Autodesk Inventor part; units mm, degrees
ref_plane "YZ Plane" through (0, 0, 0) normal (1, 0, 0) x (0, 1, 0)
ref_plane "XZ Plane" through (0, 0, 0) normal (0, 1, 0) x (-1, 0, 0)
ref_plane "XY Plane" through (0, 0, 0) normal (0, 0, 1) x (1, 0, 0)
sketch "Sketch1" plane through (0, 0, 0) normal (0, 0, 1) x (1, 0, 0)
  line L0 (0, 0) -> (0, 52)
  line L1 (0, 52) -> (3, 52)
  line L2 (3, 52) -> (3, 3)
  line L3 (3, 3) -> (52, 3)
  line L4 (52, 3) -> (52, 0)
  line L5 (52, 0) -> (0, 0)
  dimension "d0" = 3
  dimension "d1" = 3
  dimension "d2" = 52
  dimension "d3" = 52
extrude "Extrusion1" add sketch "Sketch1" along normal blind 50
sketch "Sketch2" plane through (3, 3, 0) normal (1, 0, 0) x (0, 0, -1)
  circle A0 centre (-25, 25) radius 8.8
  line L0 (0, 49) -> (-50, 49)
  line L1 (0, 0) -> (0, 49)
  circle A1 centre (-10.5, 25) radius 1.4515
  circle A2 centre (-39.5, 25) radius 1.4515
  point P0 (0, -3)
  dimension "d6" = 17.6
  dimension "d7" = 24
  dimension "d8" = 25
  dimension "d9" = 2.903
  dimension "d10" = 2.903
  dimension "d11" = 29
  dimension "d12" = 14.5
  dimension "d13" = 14.5
extrude "Extrusion2" cut sketch "Sketch2" against normal through all
sketch "Sketch3" plane through (3, 3, 0) normal (0, 1, 0) x (1, 0, 0)
  circle A0 centre (5.4515, -41.5485) radius 1.4515
  circle A1 centre (5.4515, -8.4515) radius 1.4515
  circle A2 centre (40.5485, -41.5485) radius 1.4515
  circle A3 centre (40.5485, -8.4515) radius 1.4515
  line L0 (49, -50) -> (0, -50)
  line L1 (49, 0) -> (0, 0)
  line L2 (49, 0) -> (49, -50)
  line L3 (-3, 0) -> (-3, -50)
  dimension "d16" = 2.903
  dimension "d17" = 2.903
  dimension "d18" = 2.903
  dimension "d19" = 2.903
  dimension "d20" = 7
  dimension "d21" = 7
  dimension "d22" = 7
  dimension "d23" = 7
  dimension "d24" = 7
  dimension "d25" = 7
  dimension "d26" = 7
  dimension "d27" = 7
extrude "Extrusion3" cut sketch "Sketch3" against normal through all
equation "\"BendRadius\" = Thickness"
equation "\"BendReliefWidth\" = Thickness"
equation "\"BendReliefDepth\" = 0.5 * Thickness"
equation "\"CornerReliefSize\" = 4 * Thickness"
equation "\"MinimumRemnant\" = 2 * Thickness"
equation "\"TransitionRadius\" = BendRadius"
equation "\"JacobiRadiusSize\" = BendRadius"
equation "\"GapSize\" = Thickness"
properties part number "dc motor clamp"
The model under review builds one solid part; all positions refer to its coordinate system, in mm. A direction names the side the tool comes from. Give positions to 0.01 mm unless a question says otherwise; leave off trailing zeros. Order: outer loops, then holes, each group sorted by start corner. A loop starts at its lowest first (then second) coordinate and runs counter-clockwise, first axis right, second up. Notation, with made-up numbers: M 62,-8.5 L 82,-8.5 A3 cw 82,-4.5 Z; hole C 39,-39 d7. An arc over 180 degrees is marked long. Answer in a Markdown table with one row per item. Add a question column.
1. Add section C-C on x = 8.5. State the section outline as (y, z) points.
2. For pin 1 Ø2 at (x, z) = (12.5, 20) entering from +Y; pin 2 Ø1.7 at (y, z) = (28, 10.5) entering from -X; pin 3 Ø5 at (y, z) = (40, 43.5) entering from +X, all flat-tipped, find the tip position at first contact; note any pin that passes through.
3. Add section D-D on z = 47. State the section outline as (x, y) points.
4. Mouldability with a two-part tool opening along X and no side actions: class faces 1 (the flat face through (0, 20, 19)), 2 (the cylindrical face through (42.479, 1.521, 40.568)), 3 (the flat face through (26, 0, 25)), 4 (the flat face through (3, 39, 25)) as released by +X, released by -X, zero draft, split by the parting line, or undercut.
5. Machinability: for faces 5 (the flat face through (27, 3, 25)), 6 (the cylindrical face through (1.52, 28.98, 40.57)), which of the approach directions +Z, -Z, +X, -X, +Y, -Y give a long, thin tool a straight path to every point of the face, cutting with its end or side? Answer none if there is none.
6. To check wall thickness, follow line 1 along X through (y, z) = (11, 29); line 2 along Y through (x, z) = (1, 25). State the ranges of each line that lie inside material, in increasing order.
7. Add section A-A on z = 25. State the section outline as (x, y) points.
8. Add section B-B on y = 20. State the section outline as (x, z) points.
The answers:
| question | item | result |
|---|---|---|
| 1 | outline | M 0,0 L 3,0 L 3,7 L 0,7 Z; M 0,9.9 L 3,9.9 L 3,40.1 L 0,40.1 Z; M 0,43 L 3,43 L 3,50 L 0,50 Z |
| 2 | pin 1 | y = 3 |
| 2 | pin 2 | through |
| 2 | pin 3 | x = 3 |
| 3 | outline | M 0,0 L 52,0 L 52,3 L 3,3 L 3,52 L 0,52 Z |
| 4 | face 1 | released by -X |
| 4 | face 2 | undercut |
| 4 | face 3 | zero draft |
| 4 | face 4 | released by +X |
| 5 | face 5 | +Z, -Z, +X, +Y |
| 5 | face 6 | +X, -X |
| 6 | line 1 | 0 to 3 |
| 6 | line 2 | 0 to 19.2, 36.8 to 52 |
| 7 | outline | M 0,0 L 52,0 L 52,3 L 3,3 L 3,19.2 L 0,19.2 Z; M 0,36.8 L 3,36.8 L 3,52 L 0,52 Z |
| 8 | outline | M 0,0 L 3,0 L 3,21.33 L 0,21.33 Z; M 0,28.67 L 3,28.67 L 3,50 L 0,50 Z |
